For this review, take the finished solid that the model builds, in its own axes (mm). Face numbers are marked on the shaded views. A direction names the side the tool comes from. Round coordinates to 2 decimals unless told otherwise and drop trailing zeros. Order: outer loops, then holes, each group sorted by start corner. A loop starts at its lowest first (then second) coordinate and runs counter-clockwise, first axis right, second up. Notation, with made-up numbers: (70, 30.5) -> (110, 30.5) arc R29 cw to (110, 57.5) -> close; hole circle Ø5 at (26.25, -20). An arc over 180 degrees is marked (long way). Answer in a Markdown table with one row per item.
```python
from build123d import *

# Parameters (mm, degrees)
SKETCH2_R          = 1.25
CUT_EXTRUDE1_DEPTH = 26.936075262
CHAMFER1_SIZE      = 0.2


with BuildPart() as part:
    # Sketch1 → Revolve1 (revolve)
    with BuildSketch(Plane.XY, mode=Mode.PRIVATE) as revolve1_sk:
        Polygon((0, 2.5), (0, 17.2), (-1, 17.2), (-1, 17), (-3, 17), (-3, 9), (-6, 9), (-6, 4), (-15, 4), (-15, 2.5), align=None)
    revolve(revolve1_sk.sketch.rotate(Axis((0, 0, 0), (-1, 0, 0)), 90), axis=Axis((0, 0, 0), (-1, 0, 0)))

    # Sketch2 → Cut-Extrude1 (cut, through all)
    with BuildSketch(Plane.ZY.offset(6)):
        with Locations((0, 6)):
            Circle(SKETCH2_R)
    extrude(amount=-CUT_EXTRUDE1_DEPTH, mode=Mode.SUBTRACT)

    # Chamfer1
    chamfer1_edges = [part.edges().sort_by_distance(p)[0] for p in [
        (-3, 0, 17),
        (0, 0, 17.2),
    ]]
    chamfer(chamfer1_edges, length=CHAMFER1_SIZE)


solid = part.part
```
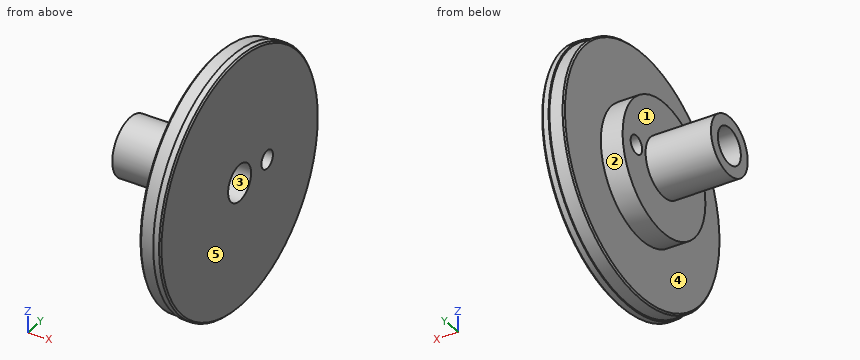
Q1. Clearance check with flat-ended pins moving along their axes: pin 1 Ø10 at (y, z) = (4.5, 3.5) entering from -X; pin 2 Ø6 at (x, y) = (-3, 8) entering from -Z; pin 3 Ø1 at (x, y) = (-6, 1) entering from -Z; pin 4 Ø8 at (x, z) = (-6, -12) entering from +Y. State where each tip first meets the part, or that it passes through.
Answer key:
| item | result |
|---|---|
| pin 1 | stops at x = -15 |
| pin 2 | stops at z = -16.25 |
| pin 3 | stops at z = -8.99 |
| pin 4 | stops at y = 14.03 |
Q2. Take a section at B-B, the plane z = 0. Write out the cut boundary in (x, y), then the cut area to 3 significant figures.
Answer key:
| item | result |
|---|---|
| outline | (-15, -4) -> (-6, -4) -> (-6, -9) -> (-3, -9) -> (-3, -16.8) -> (-2.8, -17) -> (-1, -17) -> (-1, -17.2) -> (-0.2, -17.2) -> (0, -17) -> (0, -2.5) -> (-15, -2.5) -> close; (-15, 2.5) -> (0, 2.5) -> (0, 4.75) -> (-6, 4.75) -> (-6, 4) -> (-15, 4) -> close; (-6, 7.25) -> (0, 7.25) -> (0, 17) -> (-0.2, 17.2) -> (-1, 17.2) -> (-1, 17) -> (-2.8, 17) -> (-3, 16.8) -> (-3, 9) -> (-6, 9) -> close |
| area | 138 mm^2 |
Q3. Tool access review of the marked faces 4 and 5: name each direction out of +Z, -Z, +X, -X, +Y, -Y from which nothing blocks a thin tool from reaching the whole face with its end or side.
Answer key:
| item | result |
|---|---|
| face 4 | -X |
| face 5 | +Z, -Z, +X, +Y, -Y |
Q4. The part is to be moulded in two halves that separate along Z. For the marked faces 1, 2 and 3, say which applies: +Z half, -Z half, draft (parallel to the pull), parting line (faces both ways), or undercut.
Answer key:
| item | result |
|---|---|
| face 1 | draft |
| face 2 | parting line |
| face 3 | undercut |
Q5. Take a section at A-A, the plane y = 0. Write out the cut boundary in (x, z).
Answer key:
| item | result |
|---|---|
| outline | (-15, -4) -> (-6, -4) -> (-6, -9) -> (-3, -9) -> (-3, -16.8) -> (-2.8, -17) -> (-1, -17) -> (-1, -17.2) -> (-0.2, -17.2) -> (0, -17) -> (0, -2.5) -> (-15, -2.5) -> close; (-15, 2.5) -> (0, 2.5) -> (0, 17) -> (-0.2, 17.2) -> (-1, 17.2) -> (-1, 17) -> (-2.8, 17) -> (-3, 16.8) -> (-3, 9) -> (-6, 9) -> (-6, 4) -> (-15, 4) -> close |
Q6. Take a section at C-C, the plane x = -9.5. Write out the cut boundary in (y, z).
Answer key:
| item | result |
|---|---|
| outline | circle Ø8 at (0, 0); hole circle Ø5 at (0, 0) |
Q7. To check wall thickness, follow probe 1 along Y at (x, z) = (-2.1, 0); probe 2 along Y at (x, z) = (-4.3, 0); probe 3 along Y at (x, z) = (-6.5, 0). State the ranges of each line that lie inside material, in increasing order.
Answer key:
| item | result |
|---|---|
| probe 1 | y = -17 to -2.5, 2.5 to 4.75, 7.25 to 17 |
| probe 2 | y = -9 to -2.5, 2.5 to 4.75, 7.25 to 9 |
| probe 3 | y = -4 to -2.5, 2.5 to 4 |
